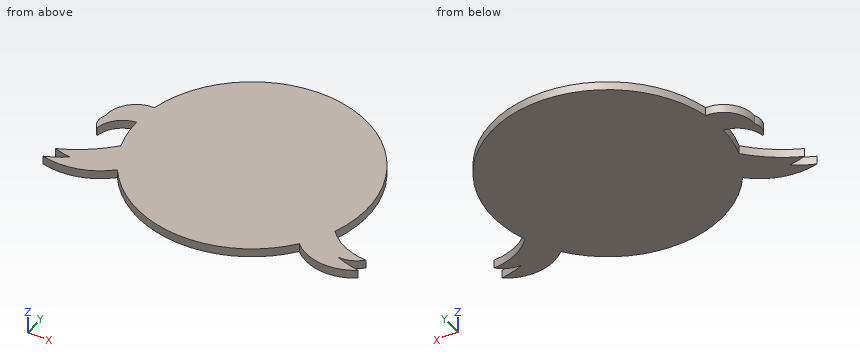
```python
from build123d import *

# Parameters (mm, degrees)
BOSS_EXTRUDE1_DEPTH = 3


with BuildPart() as part:
    # Sketch1 → Boss-Extrude1 (new body)
    with BuildSketch(Plane.XY):
        with BuildLine():
            ThreePointArc((-33.415395542, -22.883647891), (-1.332760204, -40.478065051), (31.837744667, -25.032139631))
            ThreePointArc((31.837744667, -25.032139631), (42.429569674, -29.815081636), (53.66099822, -26.828728675))
            ThreePointArc((53.66099822, -26.828728675), (49.331198922, -25.947152532), (45.137351659, -24.555756259))
            ThreePointArc((45.137351659, -24.555756259), (49.437791518, -23.866847227), (53.038636725, -21.416889589))
            ThreePointArc((53.038636725, -21.416889589), (44.73000771, -19.434385597), (37.879146269, -14.332490292))
            ThreePointArc((37.879146269, -14.332490292), (11.505540341, 38.831334531), (-39.572863934, 8.616173169))
            ThreePointArc((-39.572863934, 8.616173169), (-47.212914381, 5.371433585), (-50.134307409, -2.398004527))
            ThreePointArc((-50.134307409, -2.398004527), (-50.75248884, -5.72327668), (-49.186370781, -8.721085446))
            ThreePointArc((-49.186370781, -8.721085446), (-46.310274165, -2.976393999), (-40.499308481, -0.236669673))
            ThreePointArc((-40.499308481, -0.236669673), (-39.99258879, -6.390840467), (-38.556168915, -12.396444595))
            ThreePointArc((-38.556168915, -12.396444595), (-45.968324298, -18.925044219), (-54.579160775, -23.764068463))
            ThreePointArc((-54.579160775, -23.764068463), (-51.613504277, -24.564074489), (-48.572929157, -25))
            ThreePointArc((-48.572929157, -25), (-52.134064431, -27.12602852), (-55.899902615, -28.863884809))
            ThreePointArc((-55.899902615, -28.863884809), (-43.894548209, -28.742874568), (-33.415395542, -22.883647891))
        make_face()
    extrude(amount=BOSS_EXTRUDE1_DEPTH)


solid = part.part
```
Geometry: final body of the model. Coordinates: model frame, mm. Give positions to 0.01 mm unless a question says otherwise; leave off trailing zeros. Loops run counter-clockwise (first coordinate to the right, second up) from the corner with the lowest first, then second, coordinate; pieces in that order, holes last. Notation, with made-up numbers: (3, 41.5) -> (60, 41.5) arc R13 ccw to (60, 55.5) -> close; hole circle Ø5 at (8.25, 5.5). An arc over 180 degrees is marked (long way). Use CSV: the item, a comma, the result in double quotes.
(1) Cut plane C-C (x = -23). Output: boundary loops of the cut face in (y, z).
From the geometry:
outline,"(-33.34, 0) -> (33.34, 0) -> (33.34, 3) -> (-33.34, 3) -> close"
(2) Ray query, line 1 along X through (y, z) = (-8, 1.55); line 2 along X through (y, z) = (-7, 1.25); line 3 along Y through (x, z) = (-51, 1.2). Return the intervals inside material, ascending. Write a range as [from, to].
From the geometry:
line 1,"[-49.82, -49.06], [-39.7, 39.7]"
line 2,"[-50.39, -48.8], [-39.89, 39.89]"
line 3,"[-29.54, -26.5], [-24.68, -22.04]"
(3) First-contact query: P1, Ø1, axis at x = 42.5, z = 2.5, coming from the +Y side. Flat tip, straight axial feed; report the tip coordinate or a pass-through.
From the geometry:
P1,"y = -17.9"
(4) Cut plane D-D (y = 5). Output: boundary loops of the cut face in (x, z).
From the geometry:
outline,"(-47.55, 0) -> (40.19, 0) -> (40.19, 3) -> (-47.55, 3) -> close"
(5) Cut plane A-A (y = -5). Output: boundary loops of the cut face in (x, z).
From the geometry:
outline,"(-50.81, 0) -> (-47.9, 0) -> (-47.9, 3) -> (-50.81, 3) -> close; (-40.19, 0) -> (40.19, 0) -> (40.19, 3) -> (-40.19, 3) -> close"
(6) Cut plane B-B (z = 0.8). Output: boundary loops of the cut face in (x, y).
From the geometry:
outline,"(-55.9, -28.86) arc R24.28 ccw to (-33.42, -22.88) arc R40.5 ccw to (31.84, -25.03) arc R17.33 ccw to (53.66, -26.83) arc R37 cw to (45.14, -24.56) arc R10.01 ccw to (53.04, -21.42) arc R21.19 cw to (37.88, -14.33) arc R40.5 ccw (long way) to (-39.57, 8.62) arc R10.54 ccw to (-50.13, -2.4) arc R5.18 ccw to (-49.19, -8.72) arc R9.83 cw to (-40.5, -0.24) arc R40.5 ccw to (-38.56, -12.4) arc R47.1 cw to (-54.58, -23.76) arc R25.38 ccw to (-48.57, -25) arc R39.2 cw to start"
